Design review of the part shown in the three views and the two pictorial views. Dimensions are in mm from the part's minimum x, y and z. Coordinates: 2 decimals unless noted, no trailing zeros. Loops run counter-clockwise (first coordinate to the right, second up) from the corner with the lowest first, then second, coordinate; pieces in that order, holes last. Notation, with made-up numbers: (51, 3) -> (86, 3) arc R11 cw to (86, 12) -> close; hole circle Ø1 at (58.25, -31.75). An arc over 180 degrees is marked (long way). Use CSV: the item, a comma, the result in double quotes.
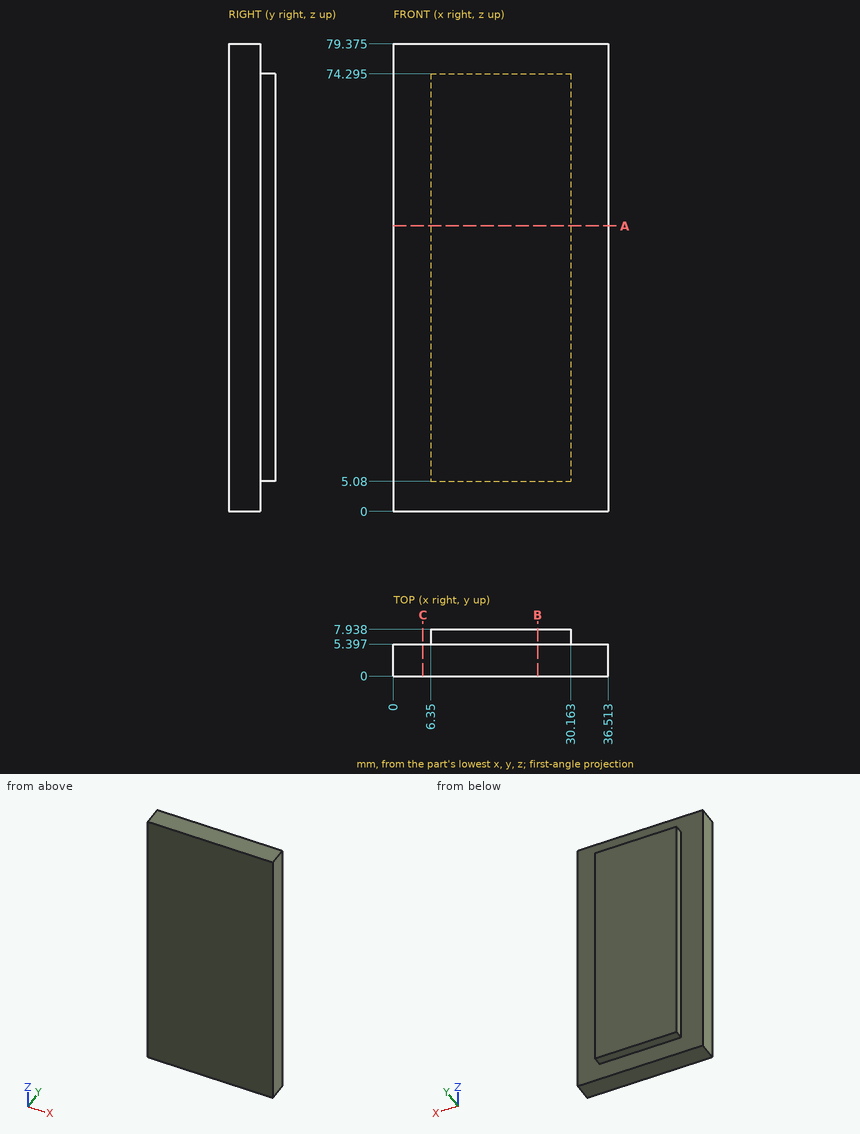
Item 1: Clearance check with flat-ended pins moving along their axes: pin 1 (3 mm diameter, centred on y = 7, z = 37, fed in from +X); pin 2 (2 mm diameter, centred on x = 21.5, y = 6.5, fed in from -Z); pin 3 (1.3 mm diameter, centred on x = 20, y = 6.5, fed in from +Z) (1 decimal). State where each tip first meets the part, or that it passes through.
Checked values:
pin 1,"x = 30.16"
pin 2,"z = 5.08"
pin 3,"z = 74.3"
Item 2: To check wall thickness, follow line 1 along X through (y, z) = (6.25, 64); line 2 along Y through (x, z) = (2, 65); line 3 along Z through (x, y) = (10, 5.5) (1 decimal). State the ranges of each line that lie inside material, in increasing order.
Checked values:
line 1,"6.35 to 30.16"
line 2,"0 to 5.4"
line 3,"5.1 to 74.3"
Item 3: Add section C-C (x = 5). Give the boundary of the cut face in (y, z) (1 decimal).
Checked values:
outline,"(0, 0) -> (5.4, 0) -> (5.4, 79.4) -> (0, 79.4) -> close"
Item 4: Add section A-A (z = 48.5). Give the boundary of the cut face in (x, y).
Checked values:
outline,"(0, 0) -> (36.51, 0) -> (36.51, 5.4) -> (30.16, 5.4) -> (30.16, 7.94) -> (6.35, 7.94) -> (6.35, 5.4) -> (0, 5.4) -> close"
Item 5: Add section B-B (x = 24.5). Give the boundary of the cut face in (y, z) (1 decimal).
Checked values:
outline,"(0, 0) -> (5.4, 0) -> (5.4, 5.1) -> (7.9, 5.1) -> (7.9, 74.3) -> (5.4, 74.3) -> (5.4, 79.4) -> (0, 79.4) -> close"
